Design review of the part built by this model. Coordinates are the model's own, in mm. Face numbers are marked on the shaded views. Give positions to 0.01 mm unless a question says otherwise; leave off trailing zeros. Write each loop counter-clockwise with the first axis right and the second up, starting at its lowest first coordinate (ties: lowest second). Pieces come first, ordered by that corner, then holes. Notation, with made-up numbers: (2, 42) -> (23, 42) arc R17 ccw to (23, 48) -> close; hole circle Ø7 at (-36.75, -39). An arc over 180 degrees is marked (long way). Put each result on its own line as item: value. Start each with the question number.
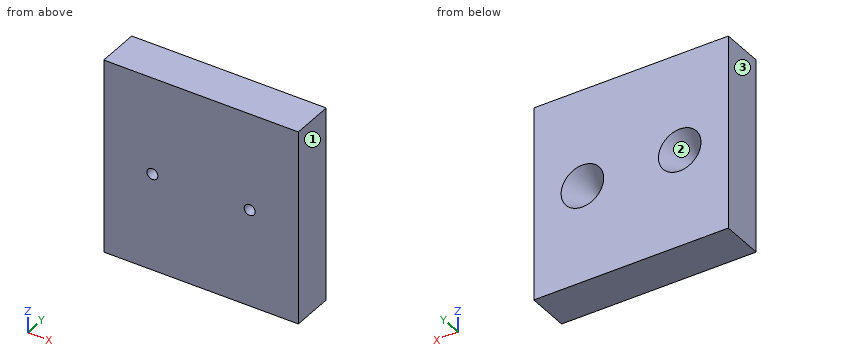
from build123d import *

# Parameters (mm, degrees)
SKETCH1_W                                            = 32
SKETCH1_H                                            = 32
BOSS_EXTRUDE1_DEPTH                                  = 3.5
CSK_FOR_M1_6_COUNTERSUNK_FLAT_HEAD_SCREW_D           = 1.8
CSK_FOR_M1_6_COUNTERSUNK_FLAT_HEAD_SCREW_CSINK_D     = 7
CSK_FOR_M1_6_COUNTERSUNK_FLAT_HEAD_SCREW_CSINK_ANGLE = 60


with BuildPart() as part:
    # Sketch1 → Boss-Extrude1 (new, symmetric)
    with BuildSketch(Plane(origin=(0, 0, 0), x_dir=(1, 0, 0), z_dir=(0, 1, 0))):
        Rectangle(SKETCH1_W, SKETCH1_H)
    extrude(amount=BOSS_EXTRUDE1_DEPTH, both=True)

    # CSK for M1.6 Countersunk Flat Head Screw1 (through all)
    with Locations(Plane(origin=(8, 3.5, 0), x_dir=(0, 0, 1), z_dir=(0, 1, 0))):
        with Locations((0, 0), (0, -16)):
            CounterSinkHole(CSK_FOR_M1_6_COUNTERSUNK_FLAT_HEAD_SCREW_D / 2, CSK_FOR_M1_6_COUNTERSUNK_FLAT_HEAD_SCREW_CSINK_D / 2, counter_sink_angle=CSK_FOR_M1_6_COUNTERSUNK_FLAT_HEAD_SCREW_CSINK_ANGLE)


solid = part.part
Q1. To check wall thickness, follow probe 1 along X at (y, z) = (-1.85, 0); probe 2 along Z at (x, y) = (-8, -2.55); probe 3 along X at (y, z) = (1.5, -0.5). State the ranges of each line that lie inside material, in increasing order. Write a range as from..to.
Q2. Take a section at C-C on y = 1.75. Give the boundary of the cut face in (x, z).
Q3. For pin 1 (1.1 mm diameter, centred on x = -8, z = 0, fed in from -Y); pin 2 (4 mm diameter, centred on x = 8.5, z = 2, fed in from +Y), all flat-tipped, find the tip position at first contact; note any pin that passes through.
Q4. Take a section at B-B on z = 0. Give the boundary of the cut face in (x, y), then the cut area to 3 significant figures.
Q5. Mouldability with a two-part tool opening along X and no side actions: class the marked faces 1, 2 and 3 as +X half, -X half, draft (parallel to the pull), parting line (faces both ways), or undercut.
Q6. Take a section at A-A on x = 8. Give the boundary of the cut face in (y, z).
Result:
1. probe 1: x = -16..-8.9, -7.1..7.1, 8.9..16
1. probe 2: z = -16..-0.9, 0.9..16
1. probe 3: x = -16..-10.29, -5.71..5.71, 10.29..16
2. outline: (-16, -16) -> (16, -16) -> (16, 16) -> (-16, 16) -> close; hole circle Ø4.98 at (-8, 0); hole circle Ø4.98 at (8, 0)
3. pin 1: passes through
3. pin 2: stops at y = 3.5
4. outline: (-16, -3.5) -> (-8.9, -3.5) -> (-8.9, -1) -> (-11.5, 3.5) -> (-16, 3.5) -> close; (-7.1, -3.5) -> (7.1, -3.5) -> (7.1, -1) -> (4.5, 3.5) -> (-4.5, 3.5) -> (-7.1, -1) -> close; (8.9, -3.5) -> (16, -3.5) -> (16, 3.5) -> (11.5, 3.5) -> (8.9, -1) -> close
4. area: 175 mm^2
5. face 1: +X half
5. face 2: undercut
5. face 3: -X half
6. outline: (-3.5, -16) -> (3.5, -16) -> (3.5, -3.5) -> (-1, -0.9) -> (-3.5, -0.9) -> close; (-3.5, 0.9) -> (-1, 0.9) -> (3.5, 3.5) -> (3.5, 16) -> (-3.5, 16) -> close
